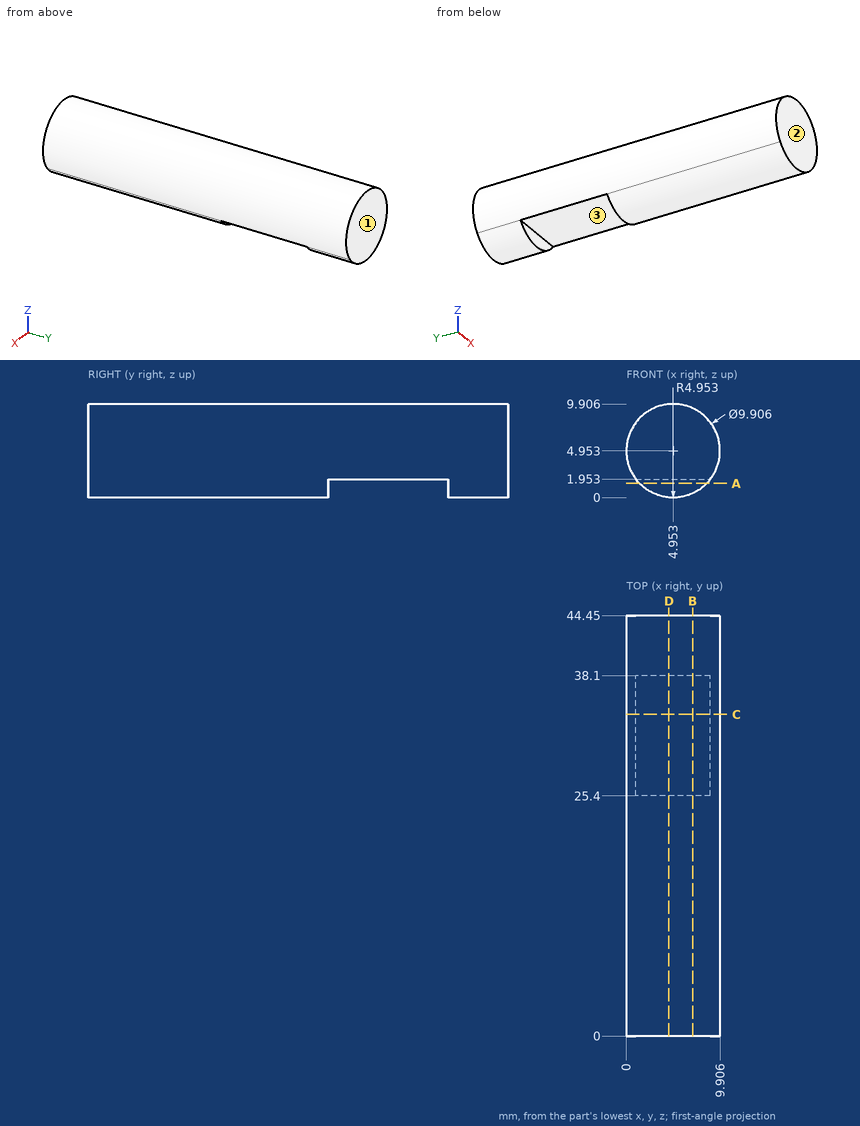
Geometry check sheet. Reference: drawing and pictorial views, mm from the part's lowest x, y, z. Round coordinates to 2 decimals unless told otherwise and drop trailing zeros. Order: outer loops, then holes, each group sorted by start corner. A loop starts at its lowest first (then second) coordinate and runs counter-clockwise, first axis right, second up. Notation, with made-up numbers: (43.5, 80) -> (95.5, 80) arc R23 cw to (95.5, 116) -> close; hole circle Ø7 at (-37.75, 79.5). An arc over 180 degrees is marked (long way). One line per item, written item: value. Start each with the question number.
Q1. Mould release check, pull along Y, two halves, no side actions. Record for the marked faces 1, 2 and 3: pulls with the +Y half, pulls with the -Y half, needs draft (parallel to the pull), parting line crosses it, or undercut.
Q2. Cross-section at B-B (x = 7). Record the boundary of the cut face in (y, z), and give its area (3 significant figures).
Q3. Cross-section at A-A (z = 1.5). Record the boundary of the cut face in (x, y), and give its area (3 significant figures).
Q4. Cross-section at D-D (x = 4.5). Record the boundary of the cut face in (y, z), and give its area (3 significant figures).
Q5. Cross-section at C-C (y = 34). Record the boundary of the cut face in (x, z), and give its area (3 significant figures).
Q6. Gauge pin test, flat ends, axial feed: pin 1 Ø4 at (x, z) = (5.5, 2.5) entering from -Y; pin 2 Ø1.5 at (x, y) = (3, 26.5) entering from +Z; pin 3 Ø2 at (x, y) = (2, 25.5) entering from +Z; pin 4 Ø4 at (x, y) = (2, 40) entering from -Z. Record the tip position at first contact, or that the pin passes through.
Q7. Thickness scan on line 1 (Y direction, x = 2, z = 1.75); line 2 (X direction, y = 13, z = 6.25). Record the ranges inside material, lowest first.
Completed:
1. face 1: pulls with the +Y half
1. face 2: pulls with the -Y half
1. face 3: undercut
2. outline: (0, 0.44) -> (25.4, 0.44) -> (25.4, 1.95) -> (38.1, 1.95) -> (38.1, 0.44) -> (44.45, 0.44) -> (44.45, 9.46) -> (0, 9.46) -> close
2. area: 382 mm²
3. outline: (1.4, 0) -> (8.5, 0) -> (8.5, 25.4) -> (1.4, 25.4) -> close; (1.4, 38.1) -> (8.5, 38.1) -> (8.5, 44.45) -> (1.4, 44.45) -> close
3. area: 225 mm²
4. outline: (0, 0.02) -> (25.4, 0.02) -> (25.4, 1.95) -> (38.1, 1.95) -> (38.1, 0.02) -> (44.45, 0.02) -> (44.45, 9.89) -> (0, 9.89) -> close
4. area: 414 mm²
5. outline: (1.01, 1.95) -> (8.89, 1.95) arc R4.95 ccw (long way) to start
5. area: 66.3 mm²
6. pin 1: stops at y = 0
6. pin 2: stops at z = 9.76
6. pin 3: stops at z = 9.5
6. pin 4: stops at z = 0.09
7. line 1: y = 0 to 25.4, 38.1 to 44.45
7. line 2: x = 0.17 to 9.73
